The listing builds one solid part. Answer for the finished solid, in the listing's coordinates (mm). Round coordinates to 2 decimals unless told otherwise and drop trailing zeros. Write each loop counter-clockwise with the first axis right and the second up, starting at its lowest first coordinate (ties: lowest second). Pieces come first, ordered by that corner, then holes. Notation, with made-up numbers: (-15, 35) - (31, 35) arc R17 cw to (31, 57) - close; hole circle Ø5 at (-30.75, -4). An arc over 180 degrees is marked (long way). Use a Markdown table: item, result. Add a question column.
1) Each of these flat-tipped pins is pushed along its axis until it touches: P1, Ø1.5, axis at x = 1, y = 65, coming from the -Z side; P2, Ø3, axis at x = -36.5, y = 50, coming from the -Z side; P3, Ø0.8, axis at y = 37.5, z = 1.5, coming from the +X side; P4, Ø0.5, axis at y = -20, z = 1.5, coming from the -X side. Where does it stop, or does it pass through?
2) A cutting plane is placed at B-B (z = 1.65). State how many separate pieces and enclosed holes the cut face has, then the cut area to 3 significant figures.
3) Find the intervals of material crossed by probe 1 along Y at (x, z) = (36.5, 0.45); probe 2 along X at (y, z) = (102, 0.3); probe 3 along X at (y, z) = (62, 1.1), in increasing order. Write a range as from..to.
4) A cutting plane is placed at A-A (y = 36.5). Give the vertices of the cut face in (x, z).
```python
from build123d import *

# Parameters (mm, degrees)
SKETCH1_W                 = 83
SKETCH1_H                 = 214
BOSS_EXTRUDE1_DEPTH       = 1
BOSS_EXTRUDE2_DEPTH       = 1
F_4_CLEARANCE_HOLE1_D     = 3.2639
F_4_CLEARANCE_HOLE1_DEPTH = 3.175
F_4_CLEARANCE_HOLE1_TIP   = 0.980574487


with BuildPart() as part:
    # Sketch1 → Boss-Extrude1 (new body)
    with BuildSketch(Plane.XY):
        Rectangle(SKETCH1_W, SKETCH1_H)
    extrude(amount=BOSS_EXTRUDE1_DEPTH)

    # Sketch2 → Boss-Extrude2 (add)
    with BuildSketch(Plane.XY.offset(1)):
        Polygon((-28.661165235, 102), (28.661165235, 102), (37.5, 93.161165235), (37.5, 82), (-37.5, 82), (-37.5, 93.161165235), align=None)
        Polygon((-28.661165235, 75.714285714), (28.661165235, 75.714285714), (37.5, 66.875450949), (37.5, 55.714285714), (-37.5, 55.714285714), (-37.5, 66.875450949), align=None)
        Polygon((-28.661165235, 49.428571429), (28.661165235, 49.428571429), (37.5, 40.589736664), (37.5, 29.428571429), (-37.5, 29.428571429), (-37.5, 40.589736664), align=None)
        Polygon((-28.661165235, 23.142857143), (28.661165235, 23.142857143), (37.5, 14.304022378), (37.5, 3.142857143), (-37.5, 3.142857143), (-37.5, 14.304022378), align=None)
        Polygon((-28.661165235, -3.142857143), (28.661165235, -3.142857143), (37.5, -11.981691908), (37.5, -23.142857143), (-37.5, -23.142857143), (-37.5, -11.981691908), align=None)
        Polygon((-28.661165235, -29.428571429), (28.661165235, -29.428571429), (37.5, -38.267406193), (37.5, -49.428571429), (-37.5, -49.428571429), (-37.5, -38.267406193), align=None)
        Polygon((-28.661165235, -55.714285714), (28.661165235, -55.714285714), (37.5, -64.553120479), (37.5, -75.714285714), (-37.5, -75.714285714), (-37.5, -64.553120479), align=None)
        Polygon((-28.661165235, -82), (28.661165235, -82), (37.5, -90.838834765), (37.5, -102), (-37.5, -102), (-37.5, -90.838834765), align=None)
    extrude(amount=BOSS_EXTRUDE2_DEPTH)

    # #4 Clearance Hole1
    with Locations(Plane.XY.offset(1)):
        with Locations((-36.5, 102), (36.5, 102), (36.5, 50), (36.5, -2), (36.5, -82), (-36.5, -82), (-36.5, -2), (-36.5, 50)):
            Hole(F_4_CLEARANCE_HOLE1_D / 2, depth=F_4_CLEARANCE_HOLE1_DEPTH)
            with Locations((0, 0, -(F_4_CLEARANCE_HOLE1_DEPTH + F_4_CLEARANCE_HOLE1_TIP / 2))):  # 118° drill point
                Cone(0, F_4_CLEARANCE_HOLE1_D / 2, F_4_CLEARANCE_HOLE1_TIP, mode=Mode.SUBTRACT)


solid = part.part
```
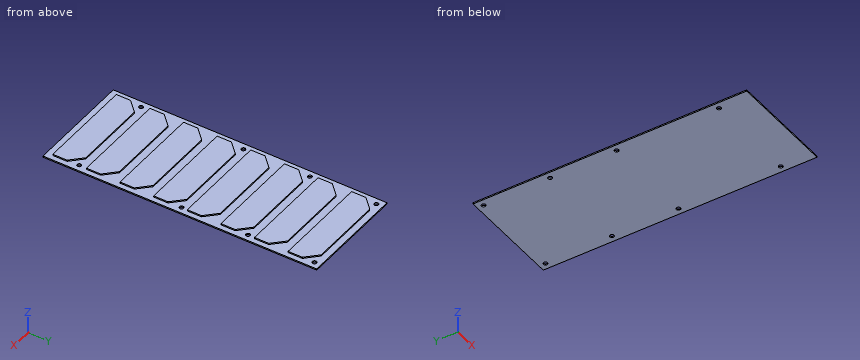
Entries:
| question | item | result |
|---|---|---|
| 1 | P1 | stops at z = 0 |
| 1 | P2 | passes through |
| 1 | P3 | stops at x = 37.5 |
| 1 | P4 | stops at x = -37.5 |
| 2 | separate pieces | 8 |
| 2 | enclosed holes | 0 |
| 2 | area | 11,400 mm² |
| 3 | probe 1 | y = -107..-83.63, -80.37..-3.63, -0.37..48.37, 51.63..100.37, 103.63..107 |
| 3 | probe 2 | x = -41.5..-38.13, -34.87..34.87, 38.13..41.5 |
| 3 | probe 3 | x = -37.5..37.5 |
| 4 | outline | (-41.5, 0) - (41.5, 0) - (41.5, 1) - (37.5, 1) - (37.5, 2) - (-37.5, 2) - (-37.5, 1) - (-41.5, 1) - close |
